Design review of the part built by this model. Coordinates are the model's own, in mm. A direction names the side the tool comes from. Give positions to 0.01 mm unless a question says otherwise; leave off trailing zeros. Write each loop counter-clockwise with the first axis right and the second up, starting at its lowest first coordinate (ties: lowest second). Pieces come first, ordered by that corner, then holes. Notation, with made-up numbers: M 30,58 L 75,58 A10 ccw 75,72 Z; hole C 66.25,-26 d5. An arc over 180 degrees is marked long. Answer in a Markdown table with one row per item.
```python
from build123d import *

# Parameters (mm, degrees)
SKETCH1_R                   = 6.35
EXTRUDE1_DEPTH              = 38.1
F_1_4_20_TAPPED_HOLE1_D     = 5.1054
F_1_4_20_TAPPED_HOLE1_DEPTH = 16.51
F_1_4_20_TAPPED_HOLE1_TIP   = 1.533816902
CHAMFER1_SIZE               = 0.396875
FILLET1_R                   = 0.79375


with BuildPart() as part:
    # Sketch1 → Extrude1 (new body)
    with BuildSketch(Plane.XY):
        with Locations(Location((0, 0, 0), (0, 0, 180))):
            Circle(SKETCH1_R)
    extrude(amount=EXTRUDE1_DEPTH)

    # 1/4-20 Tapped Hole1
    with Locations(Plane.XY.offset(38.1)):
        with Locations((0, 0)):
            Hole(F_1_4_20_TAPPED_HOLE1_D / 2, depth=F_1_4_20_TAPPED_HOLE1_DEPTH)
            with Locations((0, 0, -(F_1_4_20_TAPPED_HOLE1_DEPTH + F_1_4_20_TAPPED_HOLE1_TIP / 2))):  # 118° drill point
                Cone(0, F_1_4_20_TAPPED_HOLE1_D / 2, F_1_4_20_TAPPED_HOLE1_TIP, mode=Mode.SUBTRACT)

    # Chamfer1
    chamfer1_edges = [part.edges().sort_by_distance(p)[0] for p in [
        (6.35, 0, 38.1),
    ]]
    chamfer(chamfer1_edges, length=CHAMFER1_SIZE)

    # Fillet1
    fillet1_edges = [part.edges().sort_by_distance(p)[0] for p in [
        (6.35, 0, 0),
    ]]
    fillet(fillet1_edges, radius=FILLET1_R)


solid = part.part
```
1) The part is to be moulded in two halves that separate along X. For faces 3 (the face through (-2.93, 5.634, 18.99)), 4 (the face through (-0.1, -0.43, 20.32)), 5 (the face through (-3, 0, 38.1)), say which applies: released by +X, released by -X, zero draft, split by the parting line, or undercut.
Geometry says:
| item | result |
|---|---|
| face 3 | split by the parting line |
| face 4 | undercut |
| face 5 | zero draft |
2) To check wall thickness, follow probe 1 along Y at (x, z) = (0, 27.5); probe 2 along Z at (x, y) = (1.25, 5.5); probe 3 along Y at (x, z) = (0.25, 25.5). State the ranges of each line that lie inside material, in increasing order. Write a range as [from, to].
Geometry says:
| item | result |
|---|---|
| probe 1 | [-6.35, -2.55], [2.55, 6.35] |
| probe 2 | [0, 38.1] |
| probe 3 | [-6.35, -2.54], [2.54, 6.35] |
3) For faces 1 (the face through (-2.435, 0.767, 29.729)), 2 (the face through (0, 0, 0)), list the 3-axis set-ups (+Z, -Z, +X, -X, +Y, -Y) from which the entire face can be reached by the end or side of a thin tool; tool diameter is ignored.
Geometry says:
| item | result |
|---|---|
| face 1 | +Z |
| face 2 | -Z, +X, -X, +Y, -Y |
4) Add section A-A (z = 27). Write out the cut boundary in (x, y), and give its area (3 significant figures).
Geometry says:
| item | result |
|---|---|
| outline | C 0,0 d12.7; hole C 0,0 d5.11 |
| area | 106 mm^2 |
5) Add section B-B (z = 8). Write out the cut boundary in (x, y).
Geometry says:
| item | result |
|---|---|
| outline | C 0,0 d12.7 |
6) Insertion check: P1, Ø4, axis at x = -2.5, z = 29, coming from the -Y side; P2, Ø2, axis at y = 1.5, z = 27.5, coming from the -X side; P3, Ø3, axis at x = 0, y = 0, coming from the +Z side. Each pin has a flat end and moves straight along its axis. Give the tip position at first contact, or say it passes through.
Geometry says:
| item | result |
|---|---|
| P1 | y = -6.33 |
| P2 | x = -6.33 |
| P3 | z = 20.96 |
